Input: part model. Units: mm. Frame: model coordinates. A direction names the side the tool comes from. Give positions to 0.01 mm unless a question says otherwise; leave off trailing zeros. Write each loop counter-clockwise with the first axis right and the second up, starting at its lowest first coordinate (ties: lowest second). Pieces come first, ordered by that corner, then holes. Notation, with made-up numbers: (-17, -23) - (1, -23) arc R25 cw to (1, -7) - close; hole circle Ø4 at (14.5, -5). An arc over 180 degrees is marked (long way). Answer as CSV lines item,"result". Start each with the question number.
from build123d import *

# Parameters (mm, degrees)
F1_DEPTH = 5
F2_W     = 35
F2_H     = 155
F3_DEPTH = 5.001
F4_R     = 2.15
F5_DEPTH = 5.001


# Not quite as in the source:
# - a feature names something its author has since deleted; it is built from what else it names


with BuildPart() as f1:
    # F0 (on Top) → F1 (new body)
    with BuildSketch(Plane.XY):
        with BuildLine():
            Line((-39.5881515363, 113.7799814343), (-59.5881515363, 113.7799814343))
            Line((-59.5881515363, 113.7799814343), (-59.5881515363, -106.2200185657))
            Line((-59.5881515363, -106.2200185657), (-39.5881515363, -106.2200185657))
            ThreePointArc((-39.5881515363, -106.2200185657), (-33.7302871601, -92.0778829419), (-19.5881515363, -86.2200185657))
            Line((-19.5881515363, -86.2200185657), (120.4118484637, -86.2200185657))
            ThreePointArc((120.4118484637, -86.2200185657), (134.5539840874, -92.0778829419), (140.4118484637, -106.2200185657))
            Line((140.4118484637, -106.2200185657), (160.4118484637, -106.2200185657))
            Line((160.4118484637, -106.2200185657), (160.4118484637, 113.7799814343))
            Line((160.4118484637, 113.7799814343), (140.4118484637, 113.7799814343))
            ThreePointArc((140.4118484637, 113.7799814343), (133.0895179933, 96.1023119047), (115.4118484637, 88.7799814343))
            Line((115.4118484637, 88.7799814343), (-14.5881515363, 88.7799814343))
            ThreePointArc((-14.5881515363, 88.7799814343), (-32.265821066, 96.1023119047), (-39.5881515363, 113.7799814343))
        make_face()
    extrude(amount=F1_DEPTH)

    # F2 (on face) → F3 (cut, through all)
    with BuildSketch(Plane.XY.offset(5)):
        with Locations((50.4118484637, 1.2799814343)):
            Rectangle(F2_W, F2_H)
    extrude(amount=-F3_DEPTH, mode=Mode.SUBTRACT)

    # F4 (on face) → F5 (cut, through all)
    with BuildSketch(Plane.XY.offset(5)):
        with Locations((-49.5881515363, 103.7799814343)):
            Circle(F4_R)
        with Locations((150.4118484637, 103.7799814343)):
            Circle(F4_R)
        with Locations((50.4118484637, 83.7799814343)):
            Circle(F4_R)
        with Locations((50.4118484637, -81.2200185657)):
            Circle(F4_R)
    extrude(amount=-F5_DEPTH, mode=Mode.SUBTRACT)


solid = f1.part
1) Cut plane D-D on x = -10. Output: boundary loops of the cut face in (y, z).
2) Reachability of faces 5 (the flat face through (73, 5, 0)), 6 (the flat face through (50, -76.22, 3)), 7 (the cylindrical face through (134.398, -91.923, 2.465)), 8 (the flat face through (73, 5, 5)), 9 (the cylindrical face through (-32.07, 95.91, 2.46)) from +Z, -Z, +X, -X, +Y, -Y: full face, straight path, thin tool, end or side. Return the list, or none.
3) Cut plane C-C on z = 1.8. Output: boundary loops of the cut face in (x, y), and give its area (3 significant figures).
4) Material intervals for line 1 (X direction, y = -4.5, z = 2.95); line 2 (Y direction, x = 61.5, z = 1); line 3 (Y direction, x = 0, z = 4.1), sorted ascending. Write a range as from..to.
5) Pull-direction query (X, two-part tool) for faces 1 (the flat face through (-59.588, 5, 2)), 2 (the flat face through (32.912, 0, 3)), 3 (the cylindrical face through (-33.88, -92.23, 2.46)), 4 (the flat face through (-49, 113.78, 2)); classes: +X half, -X half, draft (parallel to the pull), parting line (faces both ways), or undercut.
6) Contact query for flat-ended pins moving along their axis: P1, Ø1, axis at x = 16, z = 4.5, coming from the +Y side; P2, Ø2.5, axis at x = 50, z = 1.5, coming from the -Y side. Output: stop coordinate, or through.
7) Cut plane A-A on y = 66.5. Output: boundary loops of the cut face in (x, z).
8) Cut plane B-B on x = 39. Output: boundary loops of the cut face in (y, z), and give its area (3 significant figures).
Numbers:
1,outline,"(-86.22, 0) - (88.78, 0) - (88.78, 5) - (-86.22, 5) - close"
2,face 5,"-Z, +X, -X, +Y, -Y"
2,face 6,"+Z, -Z"
2,face 7,"+Z, -Z, -Y"
2,face 8,"+Z, +X, -X, +Y, -Y"
2,face 9,"+Z, -Z, +Y"
3,outline,"(-59.59, -106.22) - (-39.59, -106.22) arc R20 cw to (-19.59, -86.22) - (120.41, -86.22) arc R20 cw to (140.41, -106.22) - (160.41, -106.22) - (160.41, 113.78) - (140.41, 113.78) arc R25 cw to (115.41, 88.78) - (-14.59, 88.78) arc R25 cw to (-39.59, 113.78) - (-59.59, 113.78) - close; hole circle Ø4.3 at (-49.59, 103.78); hole (32.91, -76.22) - (67.91, -76.22) - (67.91, 78.78) - (32.91, 78.78) - close; hole circle Ø4.3 at (50.41, -81.22); hole circle Ø4.3 at (50.41, 83.78); hole circle Ø4.3 at (150.41, 103.78)"
3,area,"35,300 mm²"
4,line 1,"x = -59.59..32.91, 67.91..160.41"
4,line 2,"y = -86.22..-76.22, 78.78..88.78"
4,line 3,"y = -86.22..88.78"
5,face 1,"-X half"
5,face 2,"undercut"
5,face 3,"undercut"
5,face 4,"draft"
6,P1,"stops at y = 88.78"
6,P2,"stops at y = -86.22"
7,outline,"(-59.59, 0) - (32.91, 0) - (32.91, 5) - (-59.59, 5) - close; (67.91, 0) - (160.41, 0) - (160.41, 5) - (67.91, 5) - close"
8,outline,"(-86.22, 0) - (-76.22, 0) - (-76.22, 5) - (-86.22, 5) - close; (78.78, 0) - (88.78, 0) - (88.78, 5) - (78.78, 5) - close"
8,area,"100 mm²"
